from build123d import *

# Parameters (mm, degrees)
SKETCH1_R           = 6
BOSS_EXTRUDE1_DEPTH = 15
BOSS_EXTRUDE2_DEPTH = 15
CHAMFER1_SIZE       = 2
SKETCH3_R           = 6
BOSS_EXTRUDE3_DEPTH = 15


with BuildPart() as part:
    # Sketch1 → Boss-Extrude1 (new body)
    with BuildSketch(Plane.XY):
        Circle(SKETCH1_R)
    extrude(amount=BOSS_EXTRUDE1_DEPTH)

    # Sketch2 → Boss-Extrude2 (add)
    with BuildSketch(Plane.XY.offset(15)):
        Polygon((-34.083999274, -15.270349256), (-45.136951092, -8.328867942), (-46.483233706, -4.941481314), (-45.500714563, -3.377011677), (-32.932117748, -11.270349256), (-17.560265153, -11.270349256), (-2.741776156, 0.387724819), (-13.920336004, 15.939232255), (-37.288016477, 15.939232255), (-41.885217055, 12.634724187), (-43.009602546, 14.198958718), (-42.043738714, 17.446929746), (-38.576470878, 19.939232255), (-11.869418747, 19.939232255), (2.741776156, -0.387724819), (-16.1754142, -15.270349256), align=None)
    extrude(amount=-BOSS_EXTRUDE2_DEPTH)

    # Chamfer1
    chamfer1_edges = [part.edges().sort_by_distance(p)[0] for p in [
        (-6.773577635, 12.849945977, 15),
        (-25.222944812, 19.939232255, 15),
        (-39.610475183, -11.799608599, 15),
        (-25.129706737, -15.270349256, 15),
        (-9.692346894, -10.169958865, 15),
        (-5.940891532, 0.840123687, 15),
        (5.940891532, -0.840123687, 15),
    ]]
    chamfer(chamfer1_edges, length=CHAMFER1_SIZE)

    # Sketch3 → Boss-Extrude3 (add)
    with BuildSketch(Plane(origin=(0, 0, 0), x_dir=(-1, 0, 0), z_dir=(0, 0, -1))):
        Circle(SKETCH3_R)
    extrude(amount=BOSS_EXTRUDE3_DEPTH)


solid = part.part
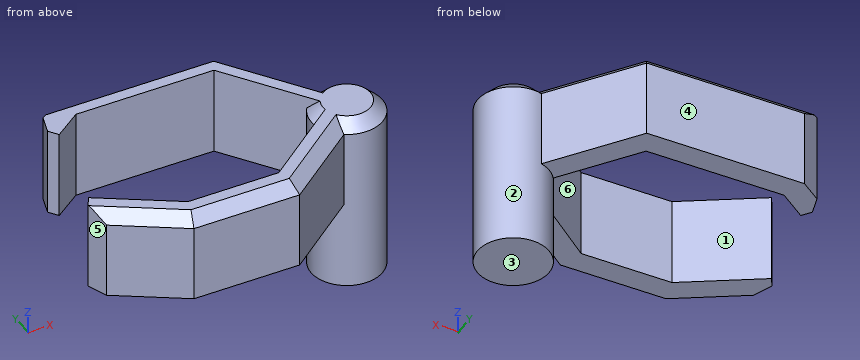
Design review of the part built by this model. Coordinates are the model's own, in mm. Face numbers are marked on the shaded views. A direction names the side the tool comes from. Coordinates: 2 decimals unless noted, no trailing zeros. Order: outer loops, then holes, each group sorted by start corner. A loop starts at its lowest first (then second) coordinate and runs counter-clockwise, first axis right, second up. Notation, with made-up numbers: (23, 51.25) -> (77, 51.25) arc R22 cw to (77, 80.25) -> close; hole circle Ø6 at (61.25, -32). An arc over 180 degrees is marked (long way). Use one line per item in the form item = value. Start each with the question number.
(1) For the marked faces 1, 2 and 3, list the 3-axis set-ups (+Z, -Z, +X, -X, +Y, -Y) from which the entire face can be reached by the end or side of a thin tool; tool diameter is ignored.
(2) Add section A-A on x = -19. State the section outline as (y, z) points, plus the area to 3 significant figures.
(3) Insertion check: pin 1 (1.5 mm diameter, centred on x = -2, y = 8.5, fed in from -Z); pin 2 (5 mm diameter, centred on x = -34, y = -8, fed in from -Z); pin 3 (10 mm diameter, centred on y = 6, z = -10.5, fed in from +X). Each pin has a flat end and moves straight along its axis. Give the tip position at first contact, or say it passes through.
(4) Add section B-B on y = 0. State the section outline as (x, z) points.
(5) For probe 1 along Y at (x, z) = (-23, 6); probe 2 along Z at (x, y) = (-26.5, 17); probe 3 along X at (y, z) = (14, 4.5), list the stretches that pass through material, from the lowest coordinate up.
(6) Add section C-C on z = -3. State the section outline as (x, y) points, plus the area to 3 significant figures.
(7) The part is to be moulded in two halves that separate along X. For the marked faces 4, 5 and 6, say which applies: +X half, -X half, draft (parallel to the pull), parting line (faces both ways), or undercut.
Answer block:
q1.face_1 = +Z, -Z
q1.face_2 = -Z
q1.face_3 = -Z, +X, -X, +Y, -Y
q2.outline = (-15.27, 0) -> (-11.27, 0) -> (-11.27, 15) -> (-13.27, 15) -> (-15.27, 13) -> close; (15.94, 0) -> (19.94, 0) -> (19.94, 13) -> (17.94, 15) -> (15.94, 15) -> close
q2.area = 116 mm²
q3.pin_1 = through
q3.pin_2 = 0
q3.pin_3 = 5.92
q4.outline = (-6, -15) -> (6, -15) -> (6, 13) -> (4, 15) -> (-4, 15) -> (-6, 13) -> close
q5.probe_1 = -15.27 to -11.27, 15.94 to 19.94
q5.probe_2 = 0 to 15
q5.probe_3 = -42.87 to -39.99, -12.53 to -7.6
q6.outline = circle Ø12 at (0, 0)
q6.area = 113 mm²
q7.face_4 = draft
q7.face_5 = -X half
q7.face_6 = undercut
